For this review, use the dimensioned drawing (mm, ordinates from the lowest corner) and the shaded views. A direction names the side the tool comes from. Coordinates: 2 decimals unless noted, no trailing zeros. Write each loop counter-clockwise with the first axis right and the second up, starting at its lowest first coordinate (ties: lowest second). Pieces come first, ordered by that corner, then holes. Notation, with made-up numbers: M 24.25,15.25 L 71.25,15.25 A27 cw 71.25,54.25 Z; hole C 38,63.5 d11. An arc over 180 degrees is marked long. Return JSON: item names as keys, results as strings. Group by question number.
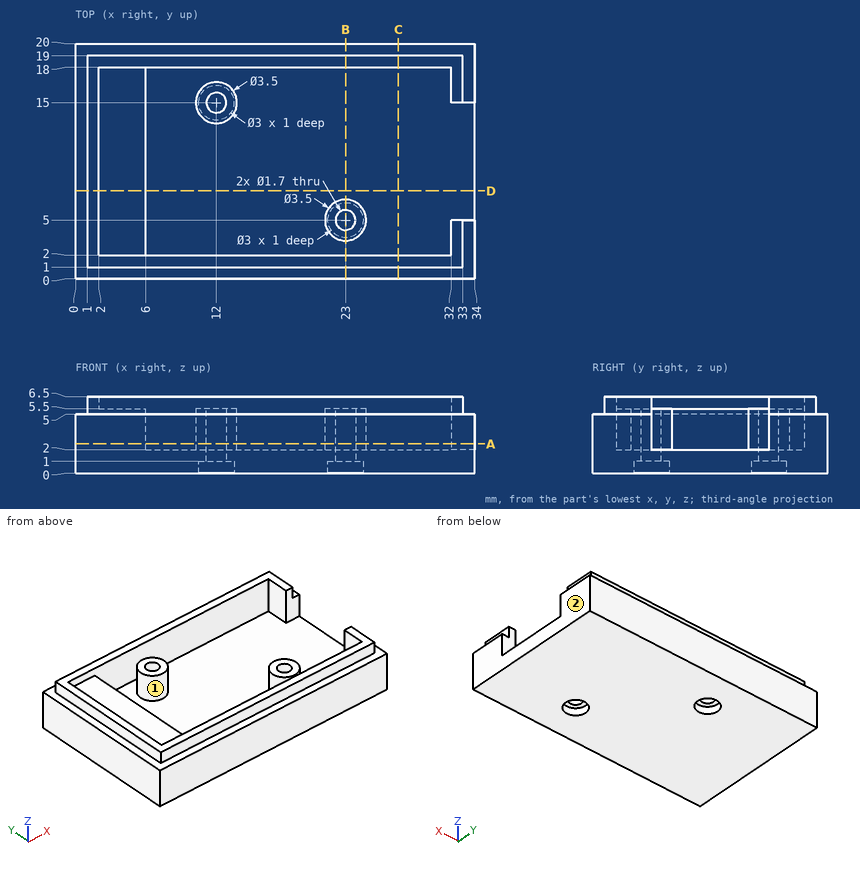
Item 1: For pin 1 (1.3 mm diameter, centred on x = 24.5, z = 5, fed in from -Y); pin 2 (1.5 mm diameter, centred on x = 12.5, y = 14.5, fed in from -Z); pin 3 (0.5 mm diameter, centred on y = 10, z = 6, fed in from +X); pin 4 (2 mm diameter, centred on x = 23, y = 5, fed in from +Z), all flat-tipped, find the tip position at first contact; note any pin that passes through.
Item 2: Add section A-A (z = 2.5). Write out the cut boundary in (x, y).
Item 3: For line 1 (Y direction, x = 17.5, z = 2.25); line 2 (Z direction, x = 13, y = 5.25); line 3 (X direction, y = 16.25, z = 4.5), list the stretches that pass through material, from the lowest coordinate up.
Item 4: Add section B-B (x = 23). Write out the cut boundary in (y, z).
Item 5: Add section D-D (y = 7.5). Write out the cut boundary in (x, z), plus the area to 3 significant figures.
Item 6: Add section C-C (x = 27.5). Write out the cut boundary in (y, z).
Item 7: Machinability: for the marked faces 1 and 2, which of the approach directions +Z, -Z, +X, -X, +Y, -Y give a long, thin tool a straight path to every point of the face, cutting with its end or side? Answer none if there is none.
Geometry check:
{
 "1": {"pin 1": "y = 0", "pin 2": "z = 1", "pin 3": "x = 2", "pin 4": "z = 5.5"},
 "2": {"outline": "M 0,0 L 34,0 L 34,5 L 32,5 L 32,2 L 6,2 L 6,18 L 32,18 L 32,15 L 34,15 L 34,20 L 0,20 Z; C 12,15 d3.5; C 23,5 d3.5; hole C 12,15 d1.7; hole C 23,5 d1.7"},
 "3": {"line 1": "0 to 2, 18 to 20", "line 2": "0 to 2", "line 3": "0 to 6, 10.78 to 13.22, 32 to 34"},
 "4": {"outline": "M 0,0 L 3.5,0 L 3.5,1 L 4.15,1 L 4.15,5.5 L 3.25,5.5 L 3.25,2 L 2,2 L 2,6.5 L 1,6.5 L 1,5 L 0,5 Z; M 5.85,1 L 6.5,1 L 6.5,0 L 20,0 L 20,5 L 19,5 L 19,6.5 L 18,6.5 L 18,2 L 6.75,2 L 6.75,5.5 L 5.85,5.5 Z"},
 "5": {"outline": "M 0,0 L 34,0 L 34,2 L 6,2 L 6,5.5 L 2,5.5 L 2,6.5 L 1,6.5 L 1,5 L 0,5 Z", "area": "89.5 mm^2"},
 "6": {"outline": "M 0,0 L 20,0 L 20,5 L 19,5 L 19,6.5 L 18,6.5 L 18,2 L 2,2 L 2,6.5 L 1,6.5 L 1,5 L 0,5 Z"},
 "7": {"face 1": "+Z", "face 2": "+Z, -Z, +X, +Y, -Y"}
}
